```python
from build123d import *

# Parameters (mm, degrees)
F1_DEPTH = 76.2
F2_W     = 14.9392048001
F2_H     = 7.519736886
F3_DEPTH = 110.691522939
F4_W     = 41.4504492655
F4_H     = 10.3266900301
F4_R     = 5.148684062
F5_DEPTH = 188


# Not quite as in the source:
# - an extrude ends at something that could not be found from the text; its depth is read off the source's solid


with BuildPart() as f1:
    # F0 (on Front) → F1 (new body)
    with BuildSketch(Plane.XZ):
        Polygon((0, 11.8811847642), (0, 0), (55.1948659122, 0), (0, 46.4719720185), (-55.4956570268, 46.4719720185), (-55.4956570268, 11.8811847642), align=None)
    extrude(amount=F1_DEPTH)

    # F2 (on face) → F3 (cut, through all)
    with BuildSketch(Plane(origin=(-55.4956570268, 0, 0), x_dir=(0, -1, 0), z_dir=(-1, 0, 0))):
        with Locations((38.1, 42.7121035755)):
            Rectangle(F2_W, F2_H)
    extrude(amount=-F3_DEPTH, mode=Mode.SUBTRACT)

    # F4 (on Top) → F5 (cut, through all)
    with BuildSketch(Plane.XY):
        with Locations((34.4696412794, -71.036654985)):
            Rectangle(F4_W, F4_H)
        with Locations((45.0900119481, -53.3901341259)):
            Circle(F4_R)
        with Locations((45.0900119481, -19.5571203102)):
            Circle(F4_R)
        with Locations((25.0240119481, -53.3901341259)):
            Circle(F4_R)
        with Locations((25.0240119481, -19.5571203102)):
            Circle(F4_R)
    extrude(amount=F5_DEPTH, mode=Mode.SUBTRACT)


solid = f1.part
```
Read the model definition and answer for the solid it produces. Units are mm, in the model's axes. A direction names the side the tool comes from. Coordinates: 2 decimals unless noted, no trailing zeros. Order: outer loops, then holes, each group sorted by start corner. A loop starts at its lowest first (then second) coordinate and runs counter-clockwise, first axis right, second up. Notation, with made-up numbers: (-23, -13.75) - (11, -13.75) arc R23 cw to (11, 3.25) - close; hole circle Ø9 at (-20, -0.5). An arc over 180 degrees is marked (long way). Answer as a JSON object with one key per item and string values. Group by question number.
Item 1: Flat-ended cylindrical pins translate along their axes: P1, Ø16.5, axis at x = 25.02, y = -19.56, coming from the +Z side; P2, Ø5, axis at y = -72, z = 25.5, coming from the +X side; P3, Ø1.5, axis at x = 20.5, z = 29, coming from the -Y side; P4, Ø8, axis at x = 25.02, y = -53.39, coming from the +Z side. Find the tip coordinate at first contact, or state that the pin passes through.
Item 2: A tool of negligible diameter and unlimited length cuts with its end or side. For faces 5 (the face through (-28, -38, 11.881)), 6 (the face through (-27, -61, 46.472)), 7 (the face through (-24, -30.63, 43)), 8 (the face through (13.744, -71, 17)), from which of +Z, -Z, +X, -X, +Y, -Y can it reach the whole face along a straight path? Write none if from no direction.
Item 3: Section C-C (x = 23) is taken. Give the vertices of the cut face in (y, z), plus the area to 3 significant figures.
Item 4: Section A-A (y = -68.5) is taken. Give the vertices of the cut face in (x, z).
Item 5: Section D-D (y = -50) is taken. Give the vertices of the cut face in (x, z).
Item 6: The mould has two halves that part along X. Classify faces 1 (the face through (-55.496, -38, 29)), 2 (the face through (39.946, -19.331, 4.973)), 3 (the face through (-21, -76.2, 29)), 4 (the face through (27.984, -37.567, 22.911)): +X half, -X half, draft (parallel to the pull), parting line (faces both ways), or undercut.
Item 7: Section B-B (z = 19) is taken. Give the vertices of the cut face in (x, y).
Item 8: Consider probe 1 along Y at (x, z) = (-45, 42.5); probe 2 along X at (y, z) = (-55.5, 17.5); probe 3 along Z at (x, y) = (-37, -3.5). Determine where each line is inside the solid, lowest interval first. Write a range as from..to.
Results are:
{
 "1": {"P1": "stops at z = 32.35", "P2": "stops at x = 13.74", "P3": "stops at y = -65.87", "P4": "passes through"},
 "2": {"face 5": "-Z, -X, +Y, -Y", "face 6": "+Z, +X, -X, +Y, -Y", "face 7": "+Z, +X, -X", "face 8": "+Z, -Z, +X, -Y"},
 "3": {"outline": "(-65.87, 0) - (-58.12, 0) - (-58.12, 27.11) - (-65.87, 27.11) - close; (-48.66, 0) - (-24.29, 0) - (-24.29, 27.11) - (-48.66, 27.11) - close; (-14.82, 0) - (0, 0) - (0, 27.11) - (-14.82, 27.11) - close", "area": "1,270 mm^2"},
 "4": {"outline": "(-55.5, 11.88) - (0, 11.88) - (0, 0) - (13.74, 0) - (13.74, 34.9) - (0, 46.47) - (-55.5, 46.47) - close"},
 "5": {"outline": "(-55.5, 11.88) - (0, 11.88) - (0, 0) - (21.15, 0) - (21.15, 28.67) - (0, 46.47) - (-55.5, 46.47) - close; (28.9, 0) - (41.21, 0) - (41.21, 11.77) - (28.9, 22.14) - close; (48.97, 0) - (55.19, 0) - (48.97, 5.25) - close"},
 "6": {"face 1": "-X half", "face 2": "undercut", "face 3": "draft", "face 4": "+X half"},
 "7": {"outline": "(-55.5, -76.2) - (13.74, -76.2) - (13.74, -65.87) - (32.63, -65.87) - (32.63, 0) - (-55.5, 0) - close; hole circle Ø10.3 at (25.02, -53.39); hole circle Ø10.3 at (25.02, -19.56)"},
 "8": {"probe 1": "y = -76.2..-45.57, -30.63..0", "probe 2": "x = -55.5..20.33, 29.72..34.41", "probe 3": "z = 11.88..46.47"}
}
